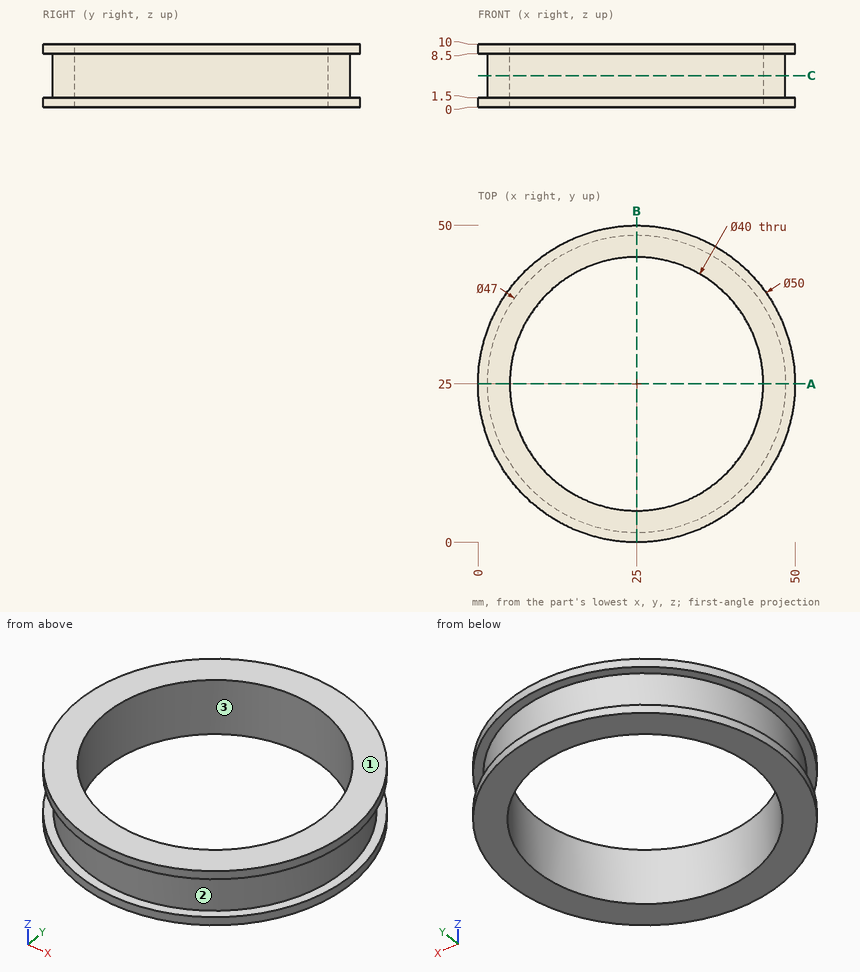
Answer from the drawing. Dimensions are ordinates in mm from the lowest x, y and z of the part. Coordinates: 2 decimals unless noted, no trailing zeros. Write each loop counter-clockwise with the first axis right and the second up, starting at its lowest first coordinate (ties: lowest second). Pieces come first, ordered by that corner, then holes. Notation, with made-up numbers: (26.5, 67.5) - (85.5, 67.5) arc R11 cw to (85.5, 77.5) - close; hole circle Ø2 at (27, -4). An arc over 180 degrees is marked (long way). Return JSON: item names as keys, results as strings. Group by question number.
Q1. Find the intervals of material crossed by line 1 along X through (y, z) = (14, 6); line 2 along Y through (x, z) = (38.5, 5.5); line 3 along X through (y, z) = (31.5, 8.75), in increasing order. Write a range as [from, to].
Q2. For a pull along X with two mould halves and no side action, classify the marked faces 1, 2 and 3 as +X half, -X half, draft (parallel to the pull), parting line (faces both ways), or undercut.
Q3. The part is cut by section A-A on y = 25. Write down the section's boundary in (x, z).
Q4. Flat-ended cylindrical pins translate along their axes: pin 1 Ø6 at (y, z) = (37.5, 5) entering from -X; pin 2 Ø2 at (x, z) = (8.5, 6) entering from +Y; pin 3 Ø1 at (x, z) = (42, 7) entering from -Y; pin 4 Ø1.5 at (x, y) = (32, 41.5) entering from +Z. Find the tip coordinate at first contact, or state that the pin passes through.
Q5. The part is cut by section C-C on z = 5. Write down the section's boundary in (x, y).
Evaluation:
{
 "1": {"line 1": "x = [4.23, 8.3], [41.7, 45.77]", "line 2": "y = [5.76, 10.24], [39.76, 44.24]", "line 3": "x = [0.86, 6.09], [43.91, 49.14]"},
 "2": {"face 1": "draft", "face 2": "parting line", "face 3": "undercut"},
 "3": {"outline": "(0, 0) - (5, 0) - (5, 10) - (0, 10) - (0, 8.5) - (1.5, 8.5) - (1.5, 1.5) - (0, 1.5) - close; (45, 0) - (50, 0) - (50, 1.5) - (48.5, 1.5) - (48.5, 8.5) - (50, 8.5) - (50, 10) - (45, 10) - close"},
 "4": {"pin 1": "stops at x = 3.51", "pin 2": "stops at y = 42.66", "pin 3": "stops at y = 8.27", "pin 4": "passes through"},
 "5": {"outline": "circle Ø47 at (25, 25); hole circle Ø40 at (25, 25)"}
}
